Work out the finished part from the listing and answer in its coordinate system (mm). A direction names the side the tool comes from. Round coordinates to 2 decimals unless told otherwise and drop trailing zeros. Loops run counter-clockwise (first coordinate to the right, second up) from the corner with the lowest first, then second, coordinate; pieces in that order, holes last.
Autodesk Inventor part; units mm, degrees
ref_plane "YZ Plane" through (0, 0, 0) normal (1, 0, 0) x (0, 1, 0)
ref_plane "XZ Plane" through (0, 0, 0) normal (0, 1, 0) x (-1, 0, 0)
ref_plane "XY Plane" through (0, 0, 0) normal (0, 0, 1) x (1, 0, 0)
sketch "Sketch1" plane through (0, 0, 0) normal (0, 1, 0) x (-1, 0, 0)
  line L0 (11.25, 6.1) -> (-11.25, 6.1)
  line L1 (-11.25, 6.1) -> (-11.25, -6.1)
  line L2 (-11.25, -6.1) -> (11.25, -6.1)
  line L3 (11.25, -6.1) -> (11.25, 6.1)
  line L4 (11.25, 6.1) -> (-11.25, -6.1) construction
  line L5 (-11.25, 6.1) -> (11.25, -6.1) construction
  point P0 (0, 0)
  dimension "d0" = 22.5
  dimension "d1" = 12.2
extrude "Extrusion1" add sketch "Sketch1" along normal blind 16
sketch "Sketch2" plane through (0, 16, 0) normal (0, 1, 0) x (1, 0, 0)
  line L0 (11.25, -6.1) -> (11.25, 6.1) construction
  line L1 (11.25, 6.1) -> (-11.25, 6.1)
  line L2 (-11.25, 6.1) -> (-11.25, -6.1) construction
  line L3 (-11.25, -6.1) -> (11.25, -6.1)
  line L4 (11.25, 6.1) -> (-11.25, 6.1)
  line L5 (-11.25, 6.1) -> (-16.1, 6.1)
  line L6 (-16.1, 6.1) -> (-16.1, -6.1)
  line L7 (-11.25, 6.1) -> (-11.25, -6.1)
  line L8 (-16.1, -6.1) -> (-11.25, -6.1)
  line L9 (11.25, -6.1) -> (11.25, 6.1)
  line L10 (11.25, -6.1) -> (16.1, -6.1)
  line L11 (16.1, -6.1) -> (16.1, 6.1)
  line L12 (16.1, 6.1) -> (11.25, 6.1)
  circle A0 centre (-14.1, 0) radius 1.4
  circle A1 centre (14.1, 0) radius 1.4
  line L13 (-11.25, -6.1) -> (11.25, -6.1) construction
  line L14 (0, -6.1) -> (0, 6.1) construction
  point P0 (0, 0)
  dimension "d5" = 32.2
  dimension "d6" = 2.8
  dimension "d7" = 2.8
  dimension "d8" = 31
extrude "Extrusion2" add sketch "Sketch2" along normal blind 2.5
sketch "Sketch3" plane through (0, 18.5, 0) normal (0, 1, 0) x (1, 0, 0)
  line L0 (11.25, -6.1) -> (11.25, 6.1)
  line L1 (-11.25, -6.1) -> (11.25, -6.1)
  line L2 (-11.25, 6.1) -> (-11.25, -6.1)
  line L3 (11.25, 6.1) -> (-11.25, 6.1)
  point P0 (0, 0)
extrude "Extrusion3" add sketch "Sketch3" along normal blind 4.2
sketch "Sketch4" plane through (0, 22.7, 0) normal (0, 1, 0) x (1, 0, 0)
  arc A0 (-5.15, 6.1) -> (0.295, -2.75) centre (-5.15, 0) ccw
  arc A1 (0.2987, 2.7426) -> (0.5, -2.75) centre (0.5, 0) ccw construction
  line L0 (11.25, 6.1) -> (-11.25, 6.1)
  line L1 (-11.25, 6.1) -> (-11.25, -6.1)
  line L2 (-11.25, -6.1) -> (11.25, -6.1)
  line L3 (11.25, -6.1) -> (11.25, 6.1)
  line L4 (0.295, 2.75) -> (0.5, 2.75)
  line L5 (0.5, -2.75) -> (0.295, -2.75)
  arc A2 (0.5, 2.75) -> (0.2987, 2.7426) centre (0.5, 0) ccw
  arc A3 (0.295, 2.75) -> (-5.15, 6.1) centre (-5.15, 0) ccw
  arc A4 (0.295, -2.75) -> (0.295, 2.75) centre (-5.15, 0) ccw construction
  arc A5 (0.5, -2.75) -> (0.5, 2.75) centre (0.5, 0) ccw
  point P0 (0, 0)
  dimension "d13" = 5.5
  dimension "d14" = 14.5
extrude "Extrusion4" add sketch "Sketch4" along normal blind 4 contours A3 L4 A5 L5 A0
sketch "Sketch5" plane through (0, 26.7, 0) normal (0, 1, 0) x (1, 0, 0)
  circle A0 centre (-5.15, 0) radius 2.5
  arc A1 (0.295, 2.75) -> (0.295, -2.75) centre (-5.15, 0) ccw
  point P0 (0, 0)
  dimension "d17" = 5
extrude "Extrusion5" add sketch "Sketch5" along normal blind 3.7
sketch "Sketch7" plane through (0, 16, 0) normal (0, -1, 0) x (1, 0, 0)
  point P0 (14.1, 0)
  point P1 (-14.1, 0)
hole "Hole2" at (14.1, 16, 0) at (-14.1, 16, 0) direction (0, 1, 0) diameter 3.4 end through all
properties part number "Motor_V1" material "Acetal Resin, Black"
1. Given pin 1 (3 mm diameter, centred on x = -8, z = -3.5, fed in from +Y); pin 2 (4.5 mm diameter, centred on x = -14.1, z = 0, fed in from -Y); pin 3 (1.5 mm diameter, centred on x = 12.5, z = 1, fed in from +Y); pin 4 (2.5 mm diameter, centred on x = 14.1, z = 0, fed in from -Y), each flat-ended and moving along its own axis, determine where each tip first touches the part or whether it passes through.
Answer key:
pin 1: stops at y = 26.7
pin 2: stops at y = 16
pin 3: stops at y = 18.5
pin 4: passes through
2. Which of the six approach directions +Z, -Z, +X, -X, +Y, -Y give full straight-line access (tool end or side, diameter ignored) to faces 1 (the face through (-10.25, 24.67, 3.35)), 2 (the face through (-12, 18.5, 0)), 3 (the face through (-11.25, 8, 0)), 4 (the face through (11.25, 21, 0))?
Answer key:
face 1: +Y
face 2: +Z, -Z, -X, +Y
face 3: +Z, -Z, -X, -Y
face 4: +Z, -Z, +X, +Y
3. Consider probe 1 along X at (y, z) = (17.6, 0); probe 2 along Z at (x, y) = (-14, 17); probe 3 along X at (y, z) = (4.5, -0.5). Determine where each line is inside the solid, lowest interval first.
Answer key:
probe 1: x = -16.1 to -15.8, -12.4 to 12.4, 15.8 to 16.1
probe 2: z = -6.1 to -1.7, 1.7 to 6.1
probe 3: x = -11.25 to 11.25
4. Find section C-C (y = 17.5). Write down the section's boundary in (x, z).
Answer key:
outline: (-16.1, -6.1) - (16.1, -6.1) - (16.1, 6.1) - (-16.1, 6.1) - close; hole circle Ø3.4 at (-14.1, 0); hole circle Ø3.4 at (14.1, 0)
5. Find section A-A (x = 14.1). Write down the section's boundary in (y, z), then the cut area to 3 significant figures.
Answer key:
outline: (16, -6.1) - (18.5, -6.1) - (18.5, -1.7) - (16, -1.7) - close; (16, 1.7) - (18.5, 1.7) - (18.5, 6.1) - (16, 6.1) - close
area: 22.0 mm2
6. Determine the mould class of faces 5 (the face through (-11.25, 21, 0)), 6 (the face through (12.414, 17.268, 0.221)), 7 (the face through (-10, 22.7, 5)) for opening direction X: +X half, -X half, draft (parallel to the pull), parting line (faces both ways), or undercut.
Answer key:
face 5: -X half
face 6: undercut
face 7: draft
7. Find section B-B (z = -0.5). Give the number of separate pieces and of enclosed holes in the cut face, then the cut area to 3 significant figures.
Answer key:
separate pieces: 3
enclosed holes: 0
area: 595 mm2
8. Find section D-D (y = 25). Write down the section's boundary in (x, z) (3 decimals).
Answer key:
outline: (-5.15, -6.1) arc R6.1 ccw to (0.295, -2.75) - (0.5, -2.75) arc R2.75 ccw to (0.5, 2.75) - (0.295, 2.75) arc R6.1 ccw (long way) to start
